Geometry: final body of the model. Coordinates: model frame, mm. A direction names the side the tool comes from. Give positions to 0.01 mm unless a question says otherwise; leave off trailing zeros. Write each loop counter-clockwise with the first axis right and the second up, starting at its lowest first coordinate (ties: lowest second). Pieces come first, ordered by that corner, then holes.
from build123d import *

# Parameters (mm, degrees)
ESQUISSE1_R             = 7.89
ESQUISSE1_R_2           = 3.885
ESQUISSE1_R_3           = 3.985
BOSS_EXTRU_1_DEPTH      = 1.58
BOSS_EXTRU_2_START      = 1.58
ESQUISSE1_3_R           = 3.885
BOSS_EXTRU_2_DEPTH      = 11.18
ESQUISSE2_R             = 3.25
BOSS_EXTRU_3_DEPTH      = 6
ENL_V_START             = -4
ESQUISSE3_R             = 3.25
ESQUISSE3_R_2           = 1.75
ENL_V_MAT_EXTRU_1_DEPTH = 1.5
CHANFREIN1_SIZE         = 1


with BuildPart() as part:
    # Esquisse1 → Boss.-Extru.1 (new body)
    # profile 1 of 11: a face of its own
    with BuildSketch(Plane(origin=(0, 0, 0), x_dir=(0, 1, 0), z_dir=(0, 0, 1))):
        with Locations((-57.907596038, 3.76712371)):
            Circle(ESQUISSE1_R)
        with Locations((-57.907596038, 3.76712371)):
            Circle(ESQUISSE1_R_2, mode=Mode.SUBTRACT)
    # profile 2 of 11: a face of its own
    with BuildSketch(Plane(origin=(0, 0, 0), x_dir=(0, 1, 0), z_dir=(0, 0, 1))):
        with Locations((-57.907596038, 3.76712371)):
            Circle(ESQUISSE1_R_2)
    # profile 3 of 11: a face of its own
    with BuildSketch(Plane(origin=(0, 0, 0), x_dir=(0, 1, 0), z_dir=(0, 0, 1))):
        with BuildLine():
            ThreePointArc((-56.301538768, 11.491933095), (-51.786979572, 8.746094895), (-50.017596038, 3.76712371))
            ThreePointArc((-50.017596038, 3.76712371), (-50.400051579, 1.340423031), (-51.510340319, -0.851016528))
            ThreePointArc((-51.510340319, -0.851016528), (-47.696280505, 4.277310952), (-43.738103365, 9.295241675))
            ThreePointArc((-43.738103365, 9.295241675), (-50.037335941, 10.293415373), (-56.301538768, 11.491933095))
        make_face()
    # profile 4 of 11: a face of its own
    with BuildSketch(Plane(origin=(0, 0, 0), x_dir=(0, 1, 0), z_dir=(0, 0, 1))):
        with BuildLine():
            ThreePointArc((-62.343020281, 10.292390891), (-59.444168438, 11.506054208), (-56.301538768, 11.491933095))
            ThreePointArc((-56.301538768, 11.491933095), (-50.037335941, 10.293415373), (-43.738103365, 9.295241675))
            ThreePointArc((-43.738103365, 9.295241675), (-25.983312523, 28.716933044), (-6.082429339, 45.932900691))
            ThreePointArc((-6.082429339, 45.932900691), (-6.808122629, 52.346571885), (-7.776764583, 58.728071842))
            ThreePointArc((-7.776764583, 58.728071842), (-7.686126552, 61.842009718), (-6.39725572, 64.678140238))
            ThreePointArc((-6.39725572, 64.678140238), (-31.994708958, 35.041699087), (-62.343020281, 10.292390891))
        make_face()
    # profile 5 of 11: a face of its own
    with BuildSketch(Plane(origin=(0, 0, 0), x_dir=(0, 1, 0), z_dir=(0, 0, 1))):
        with BuildLine():
            ThreePointArc((-7.776764583, 58.728071842), (-6.808122629, 52.346571885), (-6.082429339, 45.932900691))
            ThreePointArc((-6.082429339, 45.932900691), (-0.878320654, 49.809662788), (4.435424243, 53.534732819))
            ThreePointArc((4.435424243, 53.534732819), (-3.087690297, 52.799265283), (-7.776764583, 58.728071842))
        make_face()
    # profile 6 of 11: a face of its own
    with BuildSketch(Plane(origin=(0, 0, 0), x_dir=(0, 1, 0), z_dir=(0, 0, 1))):
        with Locations((0, 60.06)):
            Circle(ESQUISSE1_R)
        with Locations((0, 60.06)):
            Circle(ESQUISSE1_R_2, mode=Mode.SUBTRACT)
    # profile 7 of 11: a face of its own
    with BuildSketch(Plane(origin=(0, 0, 0), x_dir=(0, 1, 0), z_dir=(0, 0, 1))):
        with Locations((0, 60.06)):
            Circle(ESQUISSE1_R_2)
    # profile 8 of 11: a face of its own
    with BuildSketch(Plane(origin=(0, 0, 0), x_dir=(0, 1, 0), z_dir=(0, 0, 1))):
        with BuildLine():
            ThreePointArc((-43.738103365, 9.295241675), (-47.696280505, 4.277310952), (-51.510340319, -0.851016528))
            ThreePointArc((-51.510340319, -0.851016528), (-54.053844003, -3.117692573), (-57.315900013, -4.100658431))
            ThreePointArc((-57.315900013, -4.100658431), (-29.333901967, -3.959332501), (-1.606057271, -7.724809386))
            ThreePointArc((-1.606057271, -7.724809386), (-6.520388042, -4.442593812), (-7.776764583, 1.331928158))
            ThreePointArc((-7.776764583, 1.331928158), (-7.278629827, 4.40977224), (-6.837025839, 7.496234348))
            ThreePointArc((-6.837025839, 7.496234348), (-25.32919367, 7.541846284), (-43.738103365, 9.295241675))
        make_face()
    # profile 9 of 11: a face of its own
    with BuildSketch(Plane(origin=(0, 0, 0), x_dir=(0, 1, 0), z_dir=(0, 0, 1))):
        with BuildLine():
            ThreePointArc((4.435424243, 53.534732819), (-0.878320654, 49.809662788), (-6.082429339, 45.932900691))
            ThreePointArc((-6.082429339, 45.932900691), (-5.369716255, 26.693168194), (-6.837025839, 7.496234348))
            ThreePointArc((-6.837025839, 7.496234348), (-3.712908005, 7.657586059), (-0.591696025, 7.867782141))
            ThreePointArc((-0.591696025, 7.867782141), (4.85650588, 6.218235331), (7.776764583, 1.331928158))
            ThreePointArc((7.776764583, 1.331928158), (5.336964728, 30.03), (7.776764583, 58.728071842))
            ThreePointArc((7.776764583, 58.728071842), (6.635290614, 55.790922996), (4.435424243, 53.534732819))
        make_face()
    # profile 10 of 11: a face of its own
    with BuildSketch(Plane(origin=(0, 0, 0), x_dir=(0, 1, 0), z_dir=(0, 0, 1))):
        with BuildLine():
            ThreePointArc((-0.591696025, 7.867782141), (-3.712908005, 7.657586059), (-6.837025839, 7.496234348))
            ThreePointArc((-6.837025839, 7.496234348), (-7.278629827, 4.40977224), (-7.776764583, 1.331928158))
            ThreePointArc((-7.776764583, 1.331928158), (-5.309155306, 5.836520362), (-0.591696025, 7.867782141))
        make_face()
    # profile 11 of 11: a face of its own
    with BuildSketch(Plane(origin=(0, 0, 0), x_dir=(0, 1, 0), z_dir=(0, 0, 1))):
        Circle(ESQUISSE1_R)
        with Locations(Location((0, 0, 0), (0, 0, 90))):
            Circle(ESQUISSE1_R_3, mode=Mode.SUBTRACT)
    extrude(amount=BOSS_EXTRU_1_DEPTH)

    # Esquisse1<3> → Boss.-Extru.2 (add)
    with BuildSketch(Plane(origin=(0, 0, 0), x_dir=(0, 1, 0), z_dir=(0, 0, 1)).offset(BOSS_EXTRU_2_START)):
        with Locations(Location((0, 60.06, 0), (0, 0, 90))):
            Circle(ESQUISSE1_3_R)
        with Locations(Location((-57.907596038, 3.76712371, 0), (0, 0, 90))):
            Circle(ESQUISSE1_3_R)
    extrude(amount=BOSS_EXTRU_2_DEPTH)

    # Esquisse2 → Boss.-Extru.3 (add)
    with BuildSketch(Plane.XY.offset(12.76)):
        with Locations((-3.76712371, -57.907596038)):
            Circle(ESQUISSE2_R)
        with Locations((-60.06, 0)):
            Circle(ESQUISSE2_R)
    extrude(amount=BOSS_EXTRU_3_DEPTH)

    # Esquisse3 → Enlèv. mat.-Extru.1 (cut)
    # profile 1 of 2: a face of its own
    with BuildSketch(Plane.XY.offset(18.76).offset(ENL_V_START)):
        with Locations((-60.06, 0)):
            Circle(ESQUISSE3_R)
        with Locations((-60.06, 0)):
            Circle(ESQUISSE3_R_2, mode=Mode.SUBTRACT)
    # profile 2 of 2: a face of its own
    with BuildSketch(Plane.XY.offset(18.76).offset(ENL_V_START)):
        with Locations((-3.76712371, -57.907596038)):
            Circle(ESQUISSE3_R)
        with Locations((-3.76712371, -57.907596038)):
            Circle(ESQUISSE3_R_2, mode=Mode.SUBTRACT)
    extrude(amount=ENL_V_MAT_EXTRU_1_DEPTH, mode=Mode.SUBTRACT)

    # Chanfrein1
    chanfrein1_edges = [part.edges().sort_by_distance(p)[0] for p in [
        (-7.01712371, -57.907596038, 18.76),
        (-63.31, 0, 18.76),
    ]]
    chamfer(chanfrein1_edges, length=CHANFREIN1_SIZE)


solid = part.part
Q1. Pull-direction query (X, two-part tool) for faces 4 (the cylindrical face through (-63.307, 0.143, 16.999)), 5 (the cylindrical face through (-7.53, -25.07, 0.78)), 6 (the flat face through (-2, -59, 14.76)), 7 (the cylindrical face through (-28.46, -26.247, 0.779)); classes: released by +X, released by -X, zero draft, split by the parting line, or undercut.
Filled sheet:
face 4: split by the parting line
face 5: undercut
face 6: zero draft
face 7: undercut
Q2. Section B-B on x = -38. Output: boundary loops of the cut face in (y, z), plus the area to 3 significant figures.
Filled sheet:
outline: (-29.01, 0) - (-15.84, 0) - (-15.84, 1.58) - (-29.01, 1.58) - close; (-5.52, 0) - (5.52, 0) - (5.52, 1.58) - (-5.52, 1.58) - close
area: 38.3 mm2
Q3. Ray query, line 1 along Y through (x, z) = (0, 0.85) (3 decimals); line 2 along Z through (x, y) = (-6, -20.5); line 3 along X through (y, z) = (-36.5, 1.25). Return the intervals inside material, ascending.
Filled sheet:
line 1: y = -64.84 to -3.985, 3.985 to 7.89
line 2: z = 0 to 1.58
line 3: x = -30.78 to -17.77, -8.4 to 3.62
Q4. Section C-C on z = 9. Output: boundary loops of the cut face in (x, y) (3 decimals), plus the area to 3 significant figures.
Filled sheet:
outline: circle Ø7.77 at (-60.06, 0); circle Ø7.77 at (-3.767, -57.908)
area: 94.8 mm2
Q5. Section D-D on x = -29. Output: boundary loops of the cut face in (y, z), plus the area to 3 significant figures.
Filled sheet:
outline: (-38.46, 0) - (-25.69, 0) - (-25.69, 1.58) - (-38.46, 1.58) - close; (-5.34, 0) - (5.34, 0) - (5.34, 1.58) - (-5.34, 1.58) - close
area: 37.0 mm2
Q6. Section A-A on y = 0. Output: boundary loops of the cut face in (x, z) (3 decimals), plus the area to 3 significant figures.
Filled sheet:
outline: (-67.95, 0) - (-3.985, 0) - (-3.985, 1.58) - (-56.175, 1.58) - (-56.175, 12.76) - (-56.81, 12.76) - (-56.81, 14.76) - (-58.31, 14.76) - (-58.31, 16.26) - (-56.81, 16.26) - (-56.81, 17.76) - (-57.81, 18.76) - (-62.31, 18.76) - (-63.31, 17.76) - (-63.31, 16.26) - (-61.81, 16.26) - (-61.81, 14.76) - (-63.31, 14.76) - (-63.31, 12.76) - (-63.945, 12.76) - (-63.945, 1.58) - (-67.95, 1.58) - close; (3.985, 0) - (7.89, 0) - (7.89, 1.58) - (3.985, 1.58) - close
area: 228 mm2
Q7. Access query for faces 1 (the cylindrical face through (-58.443, -0.67, 15.5)), 2 (the cylindrical face through (-4.47, -61.08, 17)), 3 (the flat face through (-4, -58, 18.76)). Directions: +Z, -Z, +X, -X, +Y, -Y. A direction counts if a zero-diameter tool reaches every point of the face in a straight line with its end or side. Return the directions, or none.
Filled sheet:
face 1: none
face 2: +Z
face 3: +Z, +X, -X, +Y, -Y
Q8. Pin query (flat end, axial travel): P1, Ø10, axis at x = -33.5, y = -29.5, coming from the -Z side; P2, Ø2, axis at y = -1, z = 11.5, coming from the +X side (3 decimals). Return the tip coordinate at first contact, or that it passes through.
Filled sheet:
P1: stops at z = 0
P2: stops at x = -56.175
